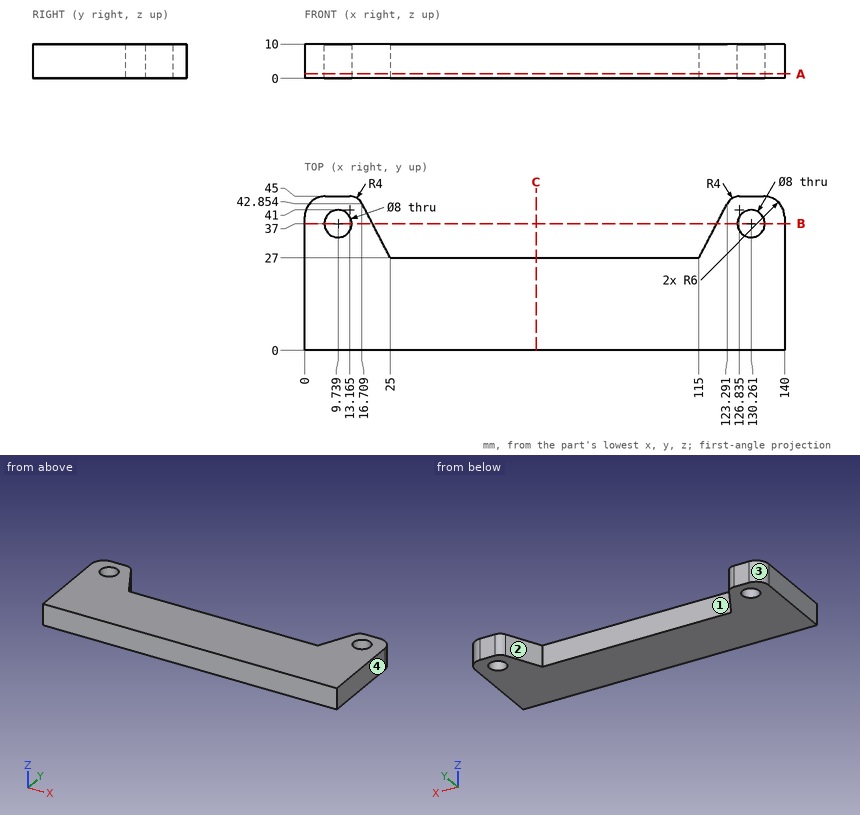
Geometry check sheet. Reference: drawing and pictorial views, mm from the part's lowest x, y, z. Coordinates: 2 decimals unless noted, no trailing zeros. Order: outer loops, then holes, each group sorted by start corner. A loop starts at its lowest first (then second) coordinate and runs counter-clockwise, first axis right, second up. Notation, with made-up numbers: M 78,77 L 120,77 A34 cw 120,107 Z; hole C 37,65 d5. An arc over 180 degrees is marked long. Return JSON: item names as keys, results as strings.
1) Release check for a two-part mould opening along X. For the marked faces 1, 2, 3 and 4 record: +X half, -X half, draft (parallel to the pull), parting line (faces both ways), or undercut.
Answer list:
{"face 1": "undercut", "face 2": "undercut", "face 3": "-X half", "face 4": "+X half"}
2) Thickness scan on L1, parallel to X at y = 39, z = 6.5 (1 decimal); L2, parallel to Y at x = 74.5, z = 7.75; L3, parallel to Y at x = 12, z = 1. Record the ranges inside material, lowest first. Write a range as [from, to].
Answer list:
{"L1": "[0, 6.3], [13.2, 18.7], [121.3, 126.8], [133.7, 140]", "L2": "[0, 27]", "L3": "[0, 33.7], [40.3, 45]"}
3) Gauge pin test, flat ends, axial feed: pin 1 (7 mm diameter, centred on x = 9.739, y = 37, fed in from +Z); pin 2 (6 mm diameter, centred on x = 103.5, z = 3.5, fed in from -Y); pin 3 (5 mm diameter, centred on x = 62, z = 3, fed in from +Y). Record the tip position at first contact, or that the pin passes through.
Answer list:
{"pin 1": "through", "pin 2": "y = 0", "pin 3": "y = 27"}
4) Cross-section at B-B, the plane y = 37. Record the boundary of the cut face in (x, z).
Answer list:
{"outline": "M 0,0 L 5.74,0 L 5.74,10 L 0,10 Z; M 13.74,0 L 19.77,0 L 19.77,10 L 13.74,10 Z; M 120.23,0 L 126.26,0 L 126.26,10 L 120.23,10 Z; M 134.26,0 L 140,0 L 140,10 L 134.26,10 Z"}
5) Cross-section at C-C, the plane x = 67.5. Record the boundary of the cut face in (y, z), and give its area (3 significant figures).
Answer list:
{"outline": "M 0,0 L 27,0 L 27,10 L 0,10 Z", "area": "270 mm2"}
6) Cross-section at A-A, the plane z = 1.25. Record the boundary of the cut face in (x, y) (1 decimal).
Answer list:
{"outline": "M 0,0 L 140,0 L 140,39 A6 ccw 134,45 L 126.8,45 A4 ccw 123.3,42.9 L 115,27 L 25,27 L 16.7,42.9 A4 ccw 13.2,45 L 6,45 A6 ccw 0,39 Z; hole C 9.7,37 d8; hole C 130.3,37 d8"}
